Could you check a few things on this model? Use its own coordinates, in mm. Face numbers are marked on the shaded views. A direction names the side the tool comes from. Coordinates: 2 decimals unless noted, no trailing zeros. Loops run counter-clockwise (first coordinate to the right, second up) from the corner with the lowest first, then second, coordinate; pieces in that order, holes last. Notation, with made-up numbers: (-10.5, 54) - (27.5, 54) arc R18 cw to (27.5, 85) - close; hole circle Ø3 at (-20, 59). An arc over 180 degrees is marked (long way). Use CSV: the item, a comma, the result in double quotes.
from build123d import *

# Parameters (mm, degrees)
CYLINDER006_R     = 3.5
CYLINDER006_DEPTH = 16
CYLINDER007_R     = 3
CYLINDER007_DEPTH = 9
CYLINDER008_R     = 1
CYLINDER008_DEPTH = 13
CYLINDER009_R     = 1
CYLINDER009_DEPTH = 13
CYLINDER003_R     = 2
CYLINDER003_DEPTH = 6
BOX003_W          = 22
BOX003_H          = 18
BOX003_DEPTH      = 10


with BuildPart() as cylinder006:
    # Cylinder006 → Cylinder006 (new body)
    with BuildSketch(Plane(origin=(0, 5, 5), x_dir=(0, 0, -1), z_dir=(1, 0, 0))):
        Circle(CYLINDER006_R)
    extrude(amount=CYLINDER006_DEPTH)


with BuildPart() as cylinder007:
    # Cylinder007 → Cylinder007 (new body)
    with BuildSketch(Plane(origin=(13, 13, 5), x_dir=(0, 0, -1), z_dir=(1, 0, 0))):
        Circle(CYLINDER007_R)
    extrude(amount=CYLINDER007_DEPTH)


with BuildPart() as cylinder008:
    # Cylinder008 → Cylinder008 (new body)
    with BuildSketch(Plane(origin=(0, 11, 5), x_dir=(0, 0, -1), z_dir=(1, 0, 0))):
        Circle(CYLINDER008_R)
    extrude(amount=CYLINDER008_DEPTH)


with BuildPart() as cylinder009:
    # Cylinder009 → Cylinder009 (new body)
    with BuildSketch(Plane(origin=(0, 15, 5), x_dir=(0, 0, -1), z_dir=(1, 0, 0))):
        Circle(CYLINDER009_R)
    extrude(amount=CYLINDER009_DEPTH)


with BuildPart() as body:
    # Cylinder003 → Cylinder003 (new body)
    with BuildSketch(Plane(origin=(16, 5, 5), x_dir=(0, 0, -1), z_dir=(1, 0, 0))):
        Circle(CYLINDER003_R)
    extrude(amount=CYLINDER003_DEPTH)

    # Fusion: union Cylinder006, Cylinder007, Cylinder008, Cylinder009
    add(cylinder006.part)
    add(cylinder007.part)
    add(cylinder008.part)
    add(cylinder009.part)


with BuildPart() as cut003:
    # Box003 → Box003 (new body)
    with BuildSketch(Plane.XY):
        with Locations((11, 9)):
            Rectangle(BOX003_W, BOX003_H)
    extrude(amount=BOX003_DEPTH)

    # Cut003: cut Body
    add(body.part, mode=Mode.SUBTRACT)


solid = cut003.part
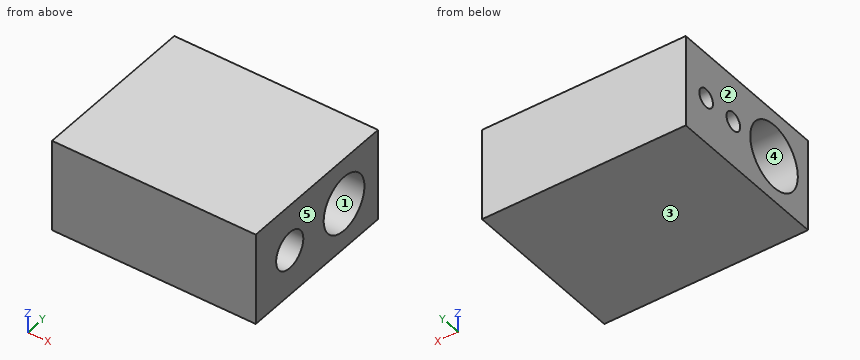
(1) Suppose I cut it at D-D (x = 15.5). Write out the boundary of the cut face in (y, z), plus the area to 3 significant figures.
Computed:
outline,"(0, 0) - (18, 0) - (18, 10) - (0, 10) - close; hole circle Ø7 at (5, 5); hole circle Ø6 at (13, 5)"
area,"113 mm²"
(2) Which directions (+Z, -Z, +X, -X, +Y, -Y) give clear straight access to the entire face, cutting with the end or side of a thin tool? Please do the marked faces 4 and 5.
Computed:
face 4,"-X"
face 5,"+Z, -Z, +X, +Y, -Y"
(3) Suppose I cut it at A-A (y = 15). Write out the boundary of the cut face in (x, z), plus the area to 3 significant figures.
Computed:
outline,"(0, 0) - (22, 0) - (22, 2.76) - (13, 2.76) - (13, 4) - (0, 4) - close; (0, 6) - (13, 6) - (13, 7.24) - (22, 7.24) - (22, 10) - (0, 10) - close"
area,"154 mm²"
(4) Please list where these lines run through material, in increasing order: line 1 (Y direction, x = 17.3, z = 5); line 2 (Y direction, x = 10.25, z = 5); line 3 (Y direction, x = 18.5, z = 4.5).
Computed:
line 1,"y = 0 to 3, 7 to 10, 16 to 18"
line 2,"y = 0 to 1.5, 8.5 to 10, 12 to 14, 16 to 18"
line 3,"y = 0 to 3.06, 6.94 to 10.04, 15.96 to 18"
(5) Will these pins go through, and if not, where does the flat tip stop? pin 1 (1.8 mm diameter, centred on y = 11, z = 5, fed in from -X); pin 2 (1.8 mm diameter, centred on y = 12, z = 4, fed in from +X).
Computed:
pin 1,"passes through"
pin 2,"stops at x = 13"
(6) Suppose I cut it at C-C (x = 3.75). Write out the boundary of the cut face in (y, z), plus the area to 3 significant figures.
Computed:
outline,"(0, 0) - (18, 0) - (18, 10) - (0, 10) - close; hole circle Ø7 at (5, 5); hole circle Ø2 at (11, 5); hole circle Ø2 at (15, 5)"
area,"135 mm²"
(7) Thinking about a two-plate mould opening in Z: for the marked faces 1, 2 and 3, which applies, +Z half, -Z half, draft (parallel to the pull), parting line (faces both ways), or undercut?
Computed:
face 1,"undercut"
face 2,"draft"
face 3,"-Z half"
(8) Suppose I cut it at B-B (z = 4.5). Write out the boundary of the cut face in (x, y), plus the area to 3 significant figures.
Computed:
outline,"(0, 0) - (22, 0) - (22, 3.06) - (16, 3.06) - (16, 1.54) - (0, 1.54) - close; (0, 8.46) - (16, 8.46) - (16, 6.94) - (22, 6.94) - (22, 10.04) - (13, 10.04) - (13, 10.13) - (0, 10.13) - close; (0, 11.87) - (13, 11.87) - (13, 14.13) - (0, 14.13) - close; (0, 15.87) - (13, 15.87) - (13, 15.96) - (22, 15.96) - (22, 18) - (0, 18) - close"
area,"164 mm²"
